Source: CAD feature listing. Evaluate the final solid. Frame: model axes, mm. Face numbers are marked on the shaded views. A direction names the side the tool comes from. Give positions to 0.01 mm unless a question says otherwise; leave off trailing zeros. Order: outer loops, then holes, each group sorted by start corner. A loop starts at its lowest first (then second) coordinate and runs counter-clockwise, first axis right, second up. Notation, with made-up numbers: (-38.75, 69) -> (-13.75, 69) arc R13 cw to (-13.75, 75) -> close; hole circle Ø5 at (57.25, 14.25). An arc over 180 degrees is marked (long way). Answer in a Markdown table with one row per item.
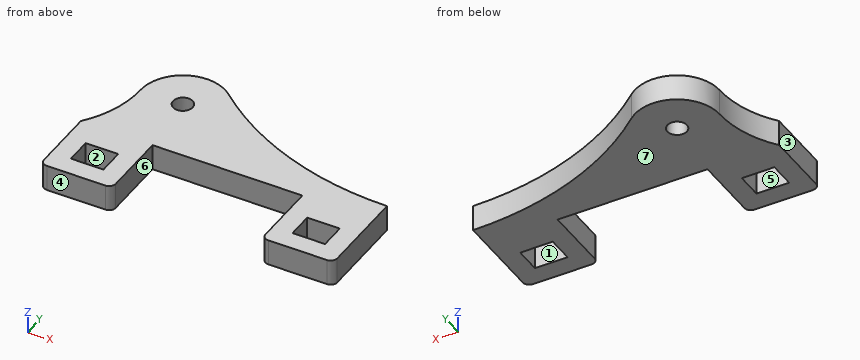
```python
from build123d import *

# Parameters (mm, degrees)
SKETCH1_W           = 5
SKETCH1_H           = 4
SKETCH1_R           = 1.5
BOSS_EXTRUDE1_DEPTH = 4
FILLET3_R           = 1


with BuildPart() as part:
    # Sketch1 → Boss-Extrude1 (new body)
    with BuildSketch(Plane.XY):
        with BuildLine():
            ThreePointArc((3.5, 10), (2.599728643, 4.702594975), (0, 0))
            Line((0, 0), (0, -11))
            Line((0, -11), (11, -11))
            Line((11, -11), (11, 0))
            Line((11, 0), (34, 0))
            Line((34, 0), (34, -11))
            Line((34, -11), (45, -11))
            Line((45, -11), (45, 3.5))
            ThreePointArc((45, 3.5), (28.59505774, 6.448232376), (14.243185079, 14.923959828))
            ThreePointArc((14.243185079, 14.923959828), (7.291744382, 15.908921349), (3.5, 10))
        make_face()
        with Locations((5.5, -6)):
            Rectangle(SKETCH1_W, SKETCH1_H, mode=Mode.SUBTRACT)
        with Locations((39.5, -6)):
            Rectangle(SKETCH1_W, SKETCH1_H, mode=Mode.SUBTRACT)
        with Locations((10, 10)):
            Circle(SKETCH1_R, mode=Mode.SUBTRACT)
    extrude(amount=BOSS_EXTRUDE1_DEPTH)

    # Fillet3
    fillet3_edges = [part.edges().sort_by_distance(p)[0] for p in [
        (45, -11, 2),
        (34, -11, 2),
        (11, -11, 2),
        (0, -11, 2),
    ]]
    fillet(fillet3_edges, radius=FILLET3_R)


solid = part.part
```
(1) Section query C-C (x = 31.5). Return the cut outline in (y, z).
A:
| item | result |
|---|---|
| outline | (0, 0) -> (5.48, 0) -> (5.48, 4) -> (0, 4) -> close |
(2) Access query for the marked faces 5, 6 and 7. Directions: +Z, -Z, +X, -X, +Y, -Y. A direction counts if a zero-diameter tool reaches every point of the face in a straight line with its end or side. Return the directions, or none.
A:
| item | result |
|---|---|
| face 5 | +Z, -Z |
| face 6 | +Z, -Z, -Y |
| face 7 | -Z, +X, -X, +Y, -Y |
(3) First-contact query: pin 1 Ø2 at (x, z) = (14.5, 1) entering from +Y; pin 2 Ø2 at (x, y) = (39, -2.5) entering from -Z; pin 3 Ø1.2 at (x, z) = (39, 2) entering from +Y. Flat tips, straight axial feed; report the tip coordinate or a pass-through.
A:
| item | result |
|---|---|
| pin 1 | stops at y = 15.48 |
| pin 2 | stops at z = 0 |
| pin 3 | stops at y = 3.96 |
(4) Pull-direction query (Y, two-part tool) for the marked faces 1, 2, 3 and 4; classes: +Y half, -Y half, draft (parallel to the pull), parting line (faces both ways), or undercut.
A:
| item | result |
|---|---|
| face 1 | undercut |
| face 2 | undercut |
| face 3 | draft |
| face 4 | -Y half |
(5) Section query B-B (y = 8). Return the cut outline in (x, z).
A:
| item | result |
|---|---|
| outline | (3.37, 0) -> (24.91, 0) -> (24.91, 4) -> (3.37, 4) -> close |
(6) Ray query, probe 1 along X at (y, z) = (-5.25, 0.35); probe 2 along Y at (x, z) = (10, 2); probe 3 along X at (y, z) = (-2, 0.9). Return the intervals inside material, ascending.
A:
| item | result |
|---|---|
| probe 1 | x = 0 to 3, 8 to 11, 34 to 37, 42 to 45 |
| probe 2 | y = -11 to 8.5, 11.5 to 16.5 |
| probe 3 | x = 0 to 11, 34 to 45 |
(7) Section query A-A (z = 2.5). Return the cut outline in (x, y), plus the area to 3 significant figures.
A:
| item | result |
|---|---|
| outline | (0, -10) arc R1 ccw to (1, -11) -> (10, -11) arc R1 ccw to (11, -10) -> (11, 0) -> (34, 0) -> (34, -10) arc R1 ccw to (35, -11) -> (44, -11) arc R1 ccw to (45, -10) -> (45, 3.5) arc R47.12 cw to (14.24, 14.92) arc R6.5 ccw to (3.5, 10) arc R16.04 cw to (0, 0) -> close; hole (3, -8) -> (8, -8) -> (8, -4) -> (3, -4) -> close; hole circle Ø3 at (10, 10); hole (37, -8) -> (42, -8) -> (42, -4) -> (37, -4) -> close |
| area | 590 mm^2 |
